Read the model definition and answer for the solid it produces. Units are mm, in the model's axes. A direction names the side the tool comes from. Round coordinates to 2 decimals unless told otherwise and drop trailing zeros. Put each result on its own line as item: value. Start each with the question number.
Q1. Each of these flat-tipped pins is pushed along its axis until it touches: pin 1 Ø8 at (y, z) = (20, -20.5) entering from -X; pin 2 Ø0.9 at (x, y) = (1.5, 17) entering from +Z; pin 3 Ø2 at (y, z) = (20.5, -1) entering from -X. Where does it stop, or does it pass through?
Q2. Find the intervals of material crossed by line 1 along X through (y, z) = (11, -3), in increasing order. Write a range as from..to.
Q3. For a pull along Y with two mould halves and no side action, classify faces 1 (the face through (68, 35, -23)), 2 (the face through (2, 10, -2)), 3 (the face through (68, 18, -46)) as pulls with the +Y half, pulls with the -Y half, needs draft (parallel to the pull), parting line crosses it, or undercut.
Q4. Which of the six approach directions +Z, -Z, +X, -X, +Y, -Y give full straight-line access (tool end or side, diameter ignored) to faces 4 (the face through (1, 17, -4)), 5 (the face through (0, 17, -23))?
from build123d import *

# Parameters (mm, degrees)
SKETCH1_W           = 138
SKETCH1_H           = 35
BOSS_EXTRUDE1_DEPTH = 46
FILLET2_R           = 1
SKETCH4_W           = 4
SKETCH4_H           = 15
CUT_EXTRUDE2_DEPTH  = 5
FILLET3_R           = 2


with BuildPart() as part:
    # Sketch1 → Boss-Extrude1 (new body)
    with BuildSketch(Plane.XY):
        with Locations((69, 17.5)):
            Rectangle(SKETCH1_W, SKETCH1_H)
    extrude(amount=-BOSS_EXTRUDE1_DEPTH)

    # Fillet2
    fillet2_edges = [part.edges().sort_by_distance(p)[0] for p in [
        (69, 35, -46),
        (69, 35, 0),
        (69, 0, 0),
        (69, 0, -46),
    ]]
    fillet(fillet2_edges, radius=FILLET2_R)

    # Sketch4 → Cut-Extrude2 (cut)
    with BuildSketch(Plane.ZY):
        with Locations((-2, 17.5)):
            Rectangle(SKETCH4_W, SKETCH4_H)
    extrude(amount=-CUT_EXTRUDE2_DEPTH, mode=Mode.SUBTRACT)

    # Fillet3
    fillet3_edges = [part.edges().sort_by_distance(p)[0] for p in [
        (5, 17.5, -4),
    ]]
    fillet(fillet3_edges, radius=FILLET3_R)


solid = part.part
Findings:
1. pin 1: x = 0
1. pin 2: z = -4
1. pin 3: x = 5
2. line 1: 4.73..138
3. face 1: pulls with the +Y half
3. face 2: undercut
3. face 3: needs draft
4. face 4: +Z, -X
4. face 5: +Z, -Z, -X, +Y, -Y
